The listing builds one solid part. Answer for the finished solid, in the listing's coordinates (mm). Face numbers are marked on the shaded views. A direction names the side the tool comes from. Round coordinates to 2 decimals unless told otherwise and drop trailing zeros. Write each loop counter-clockwise with the first axis right and the second up, starting at its lowest first coordinate (ties: lowest second). Pieces come first, ordered by that corner, then holes. Notation, with made-up numbers: (60, 59.5) - (100, 59.5) arc R12 cw to (100, 68.5) - close; hole circle Ø1 at (87.25, 74.25). An arc over 180 degrees is marked (long way). Return JSON: item names as keys, results as strings. Group by question number.
(1) Section D-D, the plane z = -2 is taken. Write down the section's boundary in (x, y), then the cut area to 3 significant figures.
(2) Section A-A, the plane y = 19.45 is taken. Write down the section's boundary in (x, z).
(3) Section C-C, the plane x = 10 is taken. Write down the section's boundary in (y, z).
(4) Section B-B, the plane z = 0 is taken. Write down the section's boundary in (x, y).
(5) Determine the mould class of the marked faces 1, 2 and 3 for opening direction Y: +Y half, -Y half, draft (parallel to the pull), parting line (faces both ways), or undercut.
(6) Find the intervals of material crossed by line 1 along Y through (x, z) = (0.85, 0); line 2 along Z through (x, y) = (17, 0.7); line 3 along Z through (x, y) = (1.6, 19.45), in increasing order. Write a range as [from, to].
(7) Each of these flat-tipped pins is pushed along its axis until it touches: pin 1 (4 mm diameter, centred on y = 18.5, z = -1, fed in from -X); pin 2 (4 mm diameter, centred on y = 10, z = 0, fed in from +X); pin 3 (3 mm diameter, centred on y = 19.45, z = 0, fed in from +X). Where does it stop, or does it pass through?
(8) Which of the six approach directions +Z, -Z, +X, -X, +Y, -Y give full straight-line access (tool end or side, diameter ignored) to the marked faces 4 and 5?
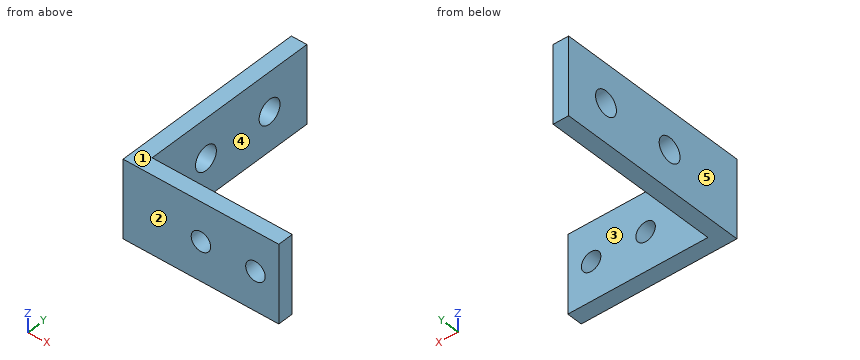
```python
from build123d import *

# Parameters (mm, degrees)
BASE_DEPTH                   = 5
M3X0_5_MOUNTHOLES_D          = 2.5
F_3_1_3_1_LIMITSWITCHHOLES_D = 3.1


with BuildPart() as part:
    # Sketch1 → Base (new body, symmetric)
    with BuildSketch(Plane.XY):
        Polygon((0, 0), (0, 25), (2, 25), (2, 2), (20, 2), (20, 0), align=None)
    extrude(amount=BASE_DEPTH, both=True)

    # M3x0.5 MountHoles (through all)
    with Locations(Plane(origin=(0, 0, 0), x_dir=(-1, 0, 0), z_dir=(0, -1, 0))):
        with Locations((-10, 0), (-17, 0)):
            Hole(M3X0_5_MOUNTHOLES_D / 2)

    # Ø3.1 (3.1) LimitSwitchHoles (through all)
    with Locations(Plane(origin=(0, 10, 0), x_dir=(0, 0, -1), z_dir=(-1, 0, 0))):
        with Locations((0, 0), (0, -9.45)):
            Hole(F_3_1_3_1_LIMITSWITCHHOLES_D / 2)


solid = part.part
```
Working result:
{
 "1": {"outline": "(0, 0) - (20, 0) - (20, 2) - (2, 2) - (2, 25) - (0, 25) - close", "area": "86.0 mm^2"},
 "2": {"outline": "(0, -5) - (2, -5) - (2, -1.55) - (0, -1.55) - close; (0, 1.55) - (2, 1.55) - (2, 5) - (0, 5) - close"},
 "3": {"outline": "(0, -5) - (2, -5) - (2, -1.25) - (0, -1.25) - close; (0, 1.25) - (2, 1.25) - (2, 5) - (0, 5) - close"},
 "4": {"outline": "(0, 0) - (8.75, 0) - (8.75, 2) - (2, 2) - (2, 8.45) - (0, 8.45) - close; (0, 11.55) - (2, 11.55) - (2, 17.9) - (0, 17.9) - close; (0, 21) - (2, 21) - (2, 25) - (0, 25) - close; (11.25, 0) - (15.75, 0) - (15.75, 2) - (11.25, 2) - close; (18.25, 0) - (20, 0) - (20, 2) - (18.25, 2) - close"},
 "5": {"face 1": "draft", "face 2": "-Y half", "face 3": "+Y half"},
 "6": {"line 1": "y = [0, 8.45], [11.55, 17.9], [21, 25]", "line 2": "z = [-5, -1.25], [1.25, 5]", "line 3": "z = [-5, -1.55], [1.55, 5]"},
 "7": {"pin 1": "stops at x = 0", "pin 2": "stops at x = 2", "pin 3": "passes through"},
 "8": {"face 4": "+Z, -Z, +X, +Y", "face 5": "+Z, -Z, -X, +Y, -Y"}
}
